Autodesk Inventor part; units mm, degrees
ref_plane "YZ Plane" through (0, 0, 0) normal (1, 0, 0) x (0, 1, 0)
ref_plane "XZ Plane" through (0, 0, 0) normal (0, 1, 0) x (-1, 0, 0)
ref_plane "XY Plane" through (0, 0, 0) normal (0, 0, 1) x (1, 0, 0)
sketch "Sketch1" plane through (0, 0, 0) normal (0, 1, 0) x (-1, 0, 0)
  line L0 (24, 8) -> (-24, 8)
  line L1 (-24, 8) -> (-24, -8)
  line L2 (-24, -8) -> (24, -8)
  line L3 (24, -8) -> (24, 8)
  point P0 (0, 0)
  dimension "d0" = 48
  dimension "d1" = 16
extrude "Extrusion1" add sketch "Sketch1" along normal blind 1
sketch "Sketch2" plane through (-24, 0, 8) normal (0, 0, 1) x (1, 0, 0)
  line L0 (0, 1) -> (1.5, 1) construction
  line L1 (0, 2.0607) -> (1.0607, 1)
  line L2 (0, 1) -> (48, 1)
  line L3 (0, 2.0607) -> (0, 1)
  line L4 (1.0607, 1) -> (2.1213, 2.0607)
  line L5 (1.0607, 1) -> (2.5607, 1) construction
  line L6 (2.1213, 2.0607) -> (3.182, 1)
  line L7 (3.182, 1) -> (4.2426, 2.0607)
  line L8 (4.2426, 2.0607) -> (5.3033, 1)
  line L9 (5.3033, 1) -> (6.364, 2.0607)
  line L10 (6.364, 2.0607) -> (7.4246, 1)
  line L11 (7.4246, 1) -> (8.4853, 2.0607)
  line L12 (7.4246, 1) -> (8.9246, 1) construction
  line L13 (8.4853, 2.0607) -> (9.5459, 1)
  line L14 (9.5459, 1) -> (10.6066, 2.0607)
  line L15 (10.6066, 2.0607) -> (11.6673, 1)
  line L16 (11.6673, 1) -> (12.7279, 2.0607)
  line L17 (12.7279, 2.0607) -> (13.7886, 1)
  line L18 (13.7886, 1) -> (14.8492, 2.0607)
  line L19 (14.8492, 2.0607) -> (15.9099, 1)
  line L20 (15.9099, 1) -> (16.9706, 2.0607)
  line L21 (16.9706, 2.0607) -> (18.0312, 1)
  line L22 (18.0312, 1) -> (19.0919, 2.0607)
  line L23 (19.0919, 2.0607) -> (20.1525, 1)
  line L24 (20.1525, 1) -> (21.2132, 2.0607)
  line L25 (21.2132, 2.0607) -> (22.2739, 1)
  line L26 (22.2739, 1) -> (23.3345, 2.0607)
  line L27 (23.3345, 2.0607) -> (24.3952, 1)
  line L28 (24.3952, 1) -> (25.4558, 2.0607)
  line L29 (25.4558, 2.0607) -> (26.5165, 1)
  line L30 (26.5165, 1) -> (27.5772, 2.0607)
  line L31 (27.5772, 2.0607) -> (28.6378, 1)
  line L32 (27.5772, 2.0607) -> (29.0772, 2.0607) construction
  line L33 (28.6378, 1) -> (29.6985, 2.0607)
  line L34 (29.6985, 2.0607) -> (30.7591, 1)
  line L35 (30.7591, 1) -> (31.8198, 2.0607)
  line L36 (31.8198, 2.0607) -> (32.8805, 1)
  line L37 (32.8805, 1) -> (33.9411, 2.0607)
  line L38 (33.9411, 2.0607) -> (35.0018, 1)
  line L39 (35.0018, 1) -> (36.0624, 2.0607)
  line L40 (36.0624, 2.0607) -> (37.1231, 1)
  line L41 (37.1231, 1) -> (38.1838, 2.0607)
  line L42 (38.1838, 2.0607) -> (39.2444, 1)
  line L43 (39.2444, 1) -> (40.3051, 2.0607)
  line L44 (40.3051, 2.0607) -> (41.3657, 1)
  line L45 (41.3657, 1) -> (42.4264, 2.0607)
  line L46 (42.4264, 2.0607) -> (43.4871, 1)
  line L47 (43.4871, 1) -> (44.5477, 2.0607)
  line L48 (44.5477, 2.0607) -> (45.6084, 1)
  line L49 (45.6084, 1) -> (46.669, 2.0607)
  line L50 (46.669, 2.0607) -> (47.7297, 1)
  line L51 (47.7297, 1) -> (48.7904, 2.0607)
  line L52 (48, 1) -> (48, 1.2703)
  line L53 (48, 0) -> (48, 1)
  line L54 (48, 1) -> (0, 1)
  point P0 (24, 0)
  point P1 (47.7297, 1)
  point P2 (47.7297, 1)
  point P3 (45.6084, 1)
  point P4 (45.6084, 1)
  point P5 (43.4871, 1)
  point P6 (43.4871, 1)
  point P7 (41.3657, 1)
  point P8 (41.3657, 1)
  point P9 (39.2444, 1)
  point P10 (39.2444, 1)
  point P11 (37.1231, 1)
  point P12 (37.1231, 1)
  point P13 (35.0018, 1)
  point P14 (35.0018, 1)
  point P15 (32.8805, 1)
  point P16 (32.8805, 1)
  point P17 (30.7591, 1)
  point P18 (30.7591, 1)
  point P19 (28.6378, 1)
  point P20 (28.6378, 1)
  point P21 (26.5165, 1)
  point P22 (26.5165, 1)
  point P23 (24.3952, 1)
  point P24 (24.3952, 1)
  point P25 (22.2739, 1)
  point P26 (22.2739, 1)
  point P27 (18.0312, 1)
  point P28 (18.0312, 1)
  point P29 (15.9099, 1)
  point P30 (15.9099, 1)
  point P31 (9.5459, 1)
  point P32 (9.5459, 1)
  dimension "d6" = 1.5
  dimension "d7" = 1.5
  dimension "d8" = 45
  dimension "d9" = 1.5
  dimension "d10" = 1.5
  dimension "d11" = 90
  dimension "d12" = 1.5
  dimension "d13" = 1.5
  dimension "d14" = 1.5
  dimension "d15" = 1.5
  dimension "d16" = 45
  dimension "d17" = 1.5
  dimension "d18" = 90
  dimension "d19" = 1.5
  dimension "d20" = 1.5
  dimension "d21" = 1.5
  dimension "d22" = 1.5
  dimension "d23" = 1.5
  dimension "d24" = 1.5
  dimension "d25" = 90
  dimension "d26" = 1.5
  dimension "d27" = 90
  dimension "d28" = 1.5
  dimension "d29" = 90
  dimension "d30" = 1.5
  dimension "d31" = 1.5
  dimension "d32" = 1.5
  dimension "d33" = 1.5
  dimension "d34" = 90
  dimension "d35" = 1.5
  dimension "d36" = 90
  dimension "d37" = 1.5
  dimension "d38" = 90
  dimension "d39" = 1.5
  dimension "d40" = 90
  dimension "d41" = 1.5
  dimension "d42" = 90
  dimension "d43" = 1.5
  dimension "d44" = 90
  dimension "d45" = 1.5
  dimension "d46" = 45
  dimension "d47" = 1.5
  dimension "d48" = 90
  dimension "d49" = 1.5
  dimension "d50" = 90
  dimension "d51" = 1.5
  dimension "d52" = 90
  dimension "d53" = 1.5
  dimension "d54" = 90
  dimension "d55" = 1.5
  dimension "d56" = 90
  dimension "d57" = 1.5
  dimension "d58" = 90
  dimension "d59" = 1.5
  dimension "d60" = 90
  dimension "d61" = 1.5
  dimension "d62" = 90
  dimension "d63" = 1.5
  dimension "d64" = 90
  dimension "d65" = 1.5
  dimension "d66" = 90
  dimension "d67" = 1.5
  dimension "d68" = 90
  dimension "d69" = 1.5
extrude "Extrusion2" add sketch "Sketch2" against normal blind 16
sketch "Sketch4" plane through (0, 0, 0) normal (0, -1, 0) x (1, 0, 0)
  line L0 (-24, 8) -> (24, 8)
  line L1 (12.5, 8) -> (-12.5, 8)
  line L2 (-12.5, 8) -> (-12.5, -8)
  line L3 (-12.5, -8) -> (12.5, -8)
  line L4 (12.5, -8) -> (12.5, 8)
  line L5 (-12.3327, 8) -> (-12.3327, -8)
  line L6 (-12.3327, 8) -> (-24, 8)
  line L7 (-24, 8) -> (-24, -8)
  line L8 (-24, -8) -> (-12.3327, -8)
  line L9 (-12.3327, -8) -> (-12.3327, 8)
  line L10 (24, 8) -> (24, -8)
  line L11 (12.5, 8) -> (24, 8)
  line L12 (24, 8) -> (24, -8)
  line L13 (24, -8) -> (12.5, -8)
  line L14 (12.5, -8) -> (12.5, 8)
  point P0 (0, 0)
  dimension "d93" = 25
  dimension "d94" = 16
extrude "Extrusion4" cut sketch "Sketch4" against normal blind 10 contours L0 L2 L8 L7 | L0 L10 L13 L4
sketch "Sketch5" plane through (0, 0, 0) normal (0, -1, 0) x (1, 0, 0)
  circle A0 centre (6.934, 5) radius 2
  circle A1 centre (-5.934, 5) radius 2
  point P0 (0, 0)
  dimension "d97" = 4
  dimension "d98" = 4
extrude "Extrusion5" cut sketch "Sketch5" against normal blind 10
mirror "Mirror1" about plane through (0, 0, 0) normal (0, 1, 0) of "Extrusion2", "Extrusion1", "Extrusion4", "Extrusion5"
properties part number "gantryTensioner2"
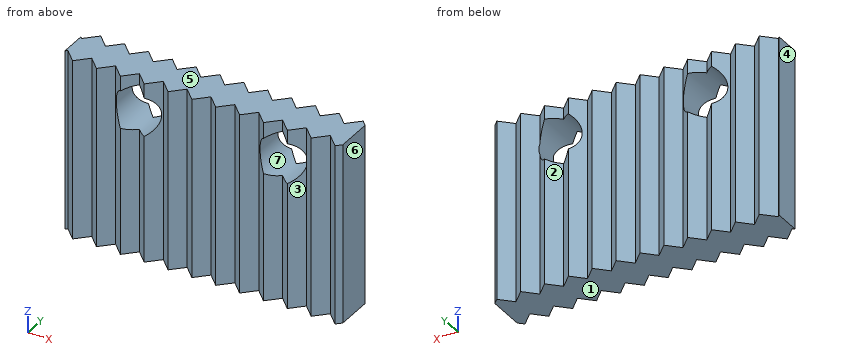
For this review, take the finished solid that the model builds, in its own axes (mm). Face numbers are marked on the shaded views. A direction names the side the tool comes from. Give positions to 0.01 mm unless a question says otherwise; leave off trailing zeros. Loops run counter-clockwise (first coordinate to the right, second up) from the corner with the lowest first, then second, coordinate; pieces in that order, holes last.
Item 1: Take a section at C-C, the plane x = -3.25. State the section outline as (y, z) points, and give its area (3 significant figures).
Item 2: For line 1 along X through (y, z) = (-0.8, 5); line 2 along X through (y, z) = (0.75, 3.75); line 3 along Z through (x, y) = (7.75, 0.7), list the stretches that pass through material, from the lowest coordinate up.
Item 3: Take a section at B-B, the plane z = 5. Give the number of separate pieces and of enclosed holes in the cut face, and give its area (3 significant figures).
Item 4: Tool access review of the marked faces 1, 2 and 3: name each direction out of +Z, -Z, +X, -X, +Y, -Y from which nothing blocks a thin tool from reaching the whole face with its end or side.
Item 5: Insertion check: pin 1 (4.5 mm diameter, centred on x = 6.934, z = 5, fed in from -Y). The pin has a flat end and moves straight along its axis. Give the tip position at first contact, or say it passes through.
Item 6: Draft analysis for pull direction X (two halves, no side actions). For the marked faces 4, 5, 6 and 7, state which applies: +X half, -X half, draft (parallel to the pull), parting line (faces both ways), or undercut.
Item 7: Take a section at D-D, the plane x = 10.5. State the section outline as (y, z) points, and give its area (3 significant figures).
Item 8: Take a section at A-A, the plane y = 0.7. State the section outline as (x, z) points, and give its area (3 significant figures).
Calculated:
1. outline: (-1.6, -8) - (1.6, -8) - (1.6, 8) - (-1.6, 8) - close
1. area: 51.1 mm2
2. line 1: x = -12.5 to -7.93, -3.93 to 4.93, 8.93 to 12.5
2. line 2: x = -12.5 to -7.5, -4.37 to 5.37, 8.5 to 12.5
2. line 3: z = -8 to 3.17, 6.83 to 8
3. separate pieces: 3
3. enclosed holes: 0
3. area: 51.8 mm2
4. face 1: -Z, +X, -X, +Y, -Y
4. face 2: +Z, -Z, +Y
4. face 3: +Z, -Z, -Y
5. pin 1: stops at y = -2.06
6. face 4: -X half
6. face 5: draft
6. face 6: +X half
6. face 7: undercut
7. outline: (-1.5, -8) - (1.5, -8) - (1.5, 8) - (-1.5, 8) - close
7. area: 48.1 mm2
8. outline: (-12.5, -8) - (12.5, -8) - (12.5, 8) - (-12.5, 8) - close; hole circle Ø4 at (-5.93, 5); hole circle Ø4 at (6.93, 5)
8. area: 375 mm2
